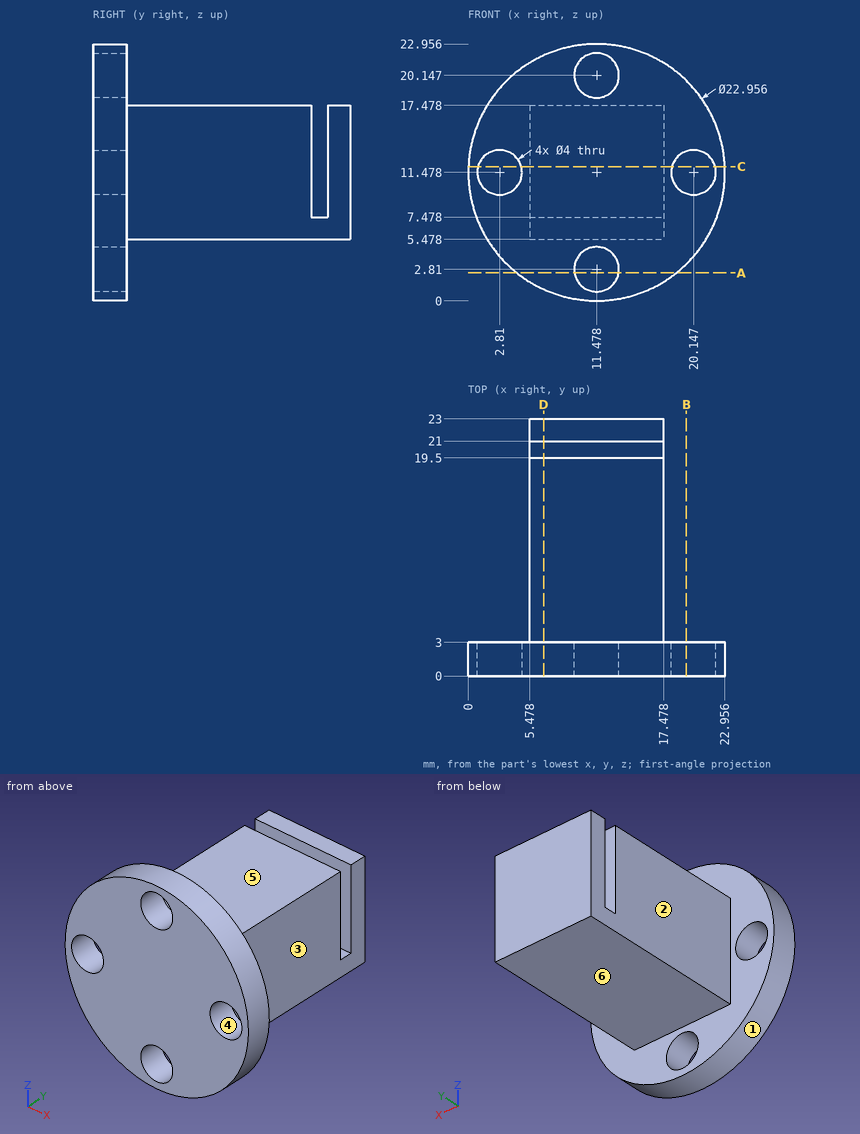
Geometry: see drawing. Coordinates: mm, zero at the bounding-box minimum. A direction names the side the tool comes from. Round coordinates to 2 decimals unless told otherwise and drop trailing zeros. Write each loop counter-clockwise with the first axis right and the second up, starting at its lowest first coordinate (ties: lowest second). Pieces come first, ordered by that corner, then holes.
1) Cut plane D-D (x = 6.75). Return the cut outline in (y, z).
2) Draft query along Z for the marked faces 4, 5 and 6. Return one class per face: pulls with the +Z half, pulls with the -Z half, needs draft (parallel to the pull), parting line crosses it, or undercut.
3) Cut plane B-B (x = 19.5). Return the cut outline in (y, z) (1 decimal).
4) Cut plane C-C (z = 12). Return the cut outline in (x, y) (1 decimal).
5) Contact query for flat-ended pins moving along their axis: P1, Ø3.5, axis at x = 13, y = 9.5, coming from the -Z side; P2, Ø3, axis at y = 4, z = 15.5, coming from the +X side; P3, Ø9.5, axis at y = 13, z = 12.5, coming from the +X side. Output: stop coordinate, or through.
6) Reachability of the marked faces 1, 2 and 3 from +Z, -Z, +X, -X, +Y, -Y: full face, straight path, thin tool, end or side. Return the list, or none.
7) Cut plane A-A (z = 2.5). Return the cut outline in (x, y).
8) Ray query, L1, parallel to Y at x = 9, z = 8; L2, parallel to Z at x = 11.75, y = 13.25; L3, parallel to Y at x = 19.75, z = 8.5. Return the intervals inside material, ascending.
Geometry says:
1. outline: (0, 1.02) - (3, 1.02) - (3, 5.48) - (23, 5.48) - (23, 17.48) - (21, 17.48) - (21, 7.48) - (19.5, 7.48) - (19.5, 17.48) - (3, 17.48) - (3, 21.94) - (0, 21.94) - close
2. face 4: undercut
2. face 5: pulls with the +Z half
2. face 6: pulls with the -Z half
3. outline: (0, 3.3) - (3, 3.3) - (3, 9.6) - (0, 9.6) - close; (0, 13.4) - (3, 13.4) - (3, 19.7) - (0, 19.7) - close
4. outline: (0, 0) - (0.9, 0) - (0.9, 3) - (0, 3) - close; (4.7, 0) - (18.2, 0) - (18.2, 3) - (17.5, 3) - (17.5, 19.5) - (5.5, 19.5) - (5.5, 3) - (4.7, 3) - close; (5.5, 21) - (17.5, 21) - (17.5, 23) - (5.5, 23) - close; (22.1, 0) - (22.9, 0) - (22.9, 3) - (22.1, 3) - close
5. P1: stops at z = 5.48
5. P2: stops at x = 22.58
5. P3: stops at x = 17.48
6. face 1: +Y, -Y
6. face 2: +Z, -Z, -X, +Y
6. face 3: +Z, -Z, +X, +Y
7. outline: (4.33, 0) - (9.5, 0) - (9.5, 3) - (4.33, 3) - close; (13.45, 0) - (18.63, 0) - (18.63, 3) - (13.45, 3) - close
8. L1: y = 0 to 19.5, 21 to 23
8. L2: z = 5.48 to 17.48
8. L3: y = 0 to 3
